The model under review builds one solid part; all positions refer to its coordinate system, in mm. Face numbers are marked on the shaded views. A direction names the side the tool comes from. Round coordinates to 2 decimals unless told otherwise and drop trailing zeros. Order: outer loops, then holes, each group sorted by start corner. A loop starts at its lowest first (then second) coordinate and runs counter-clockwise, first axis right, second up.
1) Machinability: for the marked faces 5, 6, 7 and 8, which of the approach directions +Z, -Z, +X, -X, +Y, -Y give a long, thin tool a straight path to every point of the face, cutting with its end or side? Answer none if there is none.
2) Mouldability with a two-part tool opening along Y and no side actions: class the marked faces 1, 2, 3 and 4 as pulls with the +Y half, pulls with the -Y half, needs draft (parallel to the pull), parting line crosses it, or undercut.
3) Consider section C-C (z = 2). Give the number of separate pieces and of enclosed holes in the cut face, then the cut area to 3 significant figures.
4) Consider section A-A (x = 1.5). Give the boundary of the cut face in (y, z).
5) Clearance check with flat-ended pins moving along their axes: P1, Ø1.1, axis at x = -19, z = 2.5, coming from the +Y side; P2, Ø1.5, axis at x = 14, z = 3, coming from the +Y side; P3, Ø2, axis at x = 0, z = 2, coming from the -Y side. State where each tip first meets the part, or that it passes through.
6) Consider section D-D (y = -15). Give the boundary of the cut face in (x, z).
7) To check wall thickness, follow L1, parallel to X at y = -2, z = 1.2; L2, parallel to Y at x = 16.5, z = 2.3; L3, parallel to Y at x = -16.5, z = 0.65. State the ranges of each line that lie inside material, in increasing order.
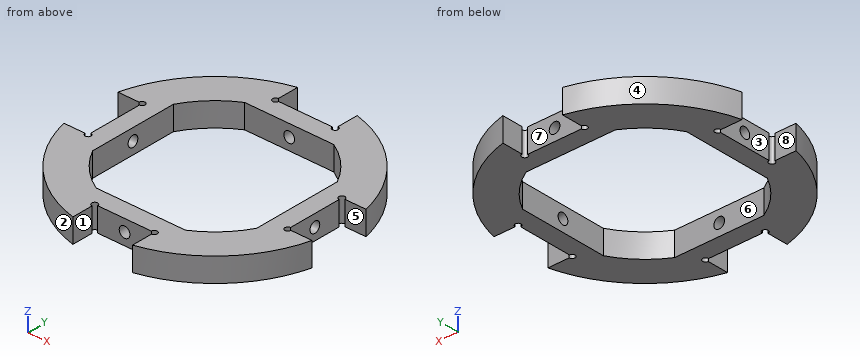
from build123d import *

# Parameters (mm, degrees)
EXTRUDE_1_DEPTH          = 4
SKETCH_2_R               = 0.9
CUT_EXTRUDE_1_DEPTH      = 43
PATTERN_CIRCULAR_1_COUNT = 4


with BuildPart() as part:
    # 草图1 → 凸台-拉伸1 (new body)
    with BuildSketch(Plane.XY):
        with BuildLine():
            Line((-4.5, 16.75), (4.5, 16.75))
            ThreePointArc((4.5, 16.75), (5.353553391, 16.396446609), (5, 17.25))
            Line((5, 17.25), (5, 20.807690886))
            ThreePointArc((5, 20.807690886), (15.132085117, 15.132085117), (20.807690886, 5))
            Line((20.807690886, 5), (17.25, 5))
            ThreePointArc((17.25, 5), (16.396446609, 5.353553391), (16.75, 4.5))
            Line((16.75, 4.5), (16.75, -4.5))
            ThreePointArc((16.75, -4.5), (16.396446609, -5.353553391), (17.25, -5))
            Line((17.25, -5), (20.807690886, -5))
            ThreePointArc((20.807690886, -5), (15.132085117, -15.132085117), (5, -20.807690886))
            Line((5, -20.807690886), (5, -17.25))
            ThreePointArc((5, -17.25), (5.353553391, -16.396446609), (4.5, -16.75))
            Line((4.5, -16.75), (-4.5, -16.75))
            ThreePointArc((-4.5, -16.75), (-5.353553391, -16.396446609), (-5, -17.25))
            Line((-5, -17.25), (-5, -20.807690886))
            ThreePointArc((-5, -20.807690886), (-15.132085117, -15.132085117), (-20.807690886, -5))
            Line((-20.807690886, -5), (-17.25, -5))
            ThreePointArc((-17.25, -5), (-16.396446609, -5.353553391), (-16.75, -4.5))
            Line((-16.75, -4.5), (-16.75, 4.5))
            ThreePointArc((-16.75, 4.5), (-16.396446609, 5.353553391), (-17.25, 5))
            Line((-17.25, 5), (-20.807690886, 5))
            ThreePointArc((-20.807690886, 5), (-15.132085117, 15.132085117), (-5, 20.807690886))
            Line((-5, 20.807690886), (-5, 17.25))
            ThreePointArc((-5, 17.25), (-5.353553391, 16.396446609), (-4.5, 16.75))
        make_face()
        with BuildLine():
            Line((-7.473954776, -13.75), (7.473954776, -13.75))
            ThreePointArc((7.473954776, -13.75), (11.066221126, -11.066221126), (13.75, -7.473954776))
            Line((13.75, -7.473954776), (13.75, 7.473954776))
            ThreePointArc((13.75, 7.473954776), (11.066221126, 11.066221126), (7.473954776, 13.75))
            Line((7.473954776, 13.75), (-7.473954776, 13.75))
            ThreePointArc((-7.473954776, 13.75), (-11.066221126, 11.066221126), (-13.75, 7.473954776))
            Line((-13.75, 7.473954776), (-13.75, -7.473954776))
            ThreePointArc((-13.75, -7.473954776), (-11.066221126, -11.066221126), (-7.473954776, -13.75))
        make_face(mode=Mode.SUBTRACT)
    extrude(amount=EXTRUDE_1_DEPTH)

    # 草图2 → 切除-拉伸1 (cut)
    with BuildSketch(Plane(origin=(0, 16.75, 0), x_dir=(1, 0, 0), z_dir=(0, 1, 0))):
        with Locations(Location((0, -2, 0), (0, 0, 180))):
            Circle(SKETCH_2_R)
    cut_extrude_1 = extrude(amount=-CUT_EXTRUDE_1_DEPTH, mode=Mode.SUBTRACT)

    # 阵列(圆周)1: 切除-拉伸1 ×4 about axis
    pattern_circular_1_axis = Axis((0, 0, 4), (0, 0, -1))
    for i in range(1, PATTERN_CIRCULAR_1_COUNT):
        add(cut_extrude_1.rotate(pattern_circular_1_axis, i * 360 / PATTERN_CIRCULAR_1_COUNT), mode=Mode.SUBTRACT)


solid = part.part
Answer below:
1. face 5: +Z, -Z, +X
1. face 6: +Z, -Z
1. face 7: +Z, -Z, +Y
1. face 8: +Z, -Z, -X
2. face 1: needs draft
2. face 2: pulls with the -Y half
2. face 3: undercut
2. face 4: pulls with the +Y half
3. separate pieces: 4
3. enclosed holes: 0
3. area: 542 mm2
4. outline: (-16.75, 0) - (-13.75, 0) - (-13.75, 4) - (-16.75, 4) - close; (13.75, 0) - (16.75, 0) - (16.75, 4) - (13.75, 4) - close
5. P1: stops at y = 10.84
5. P2: stops at y = 16.8
5. P3: stops at y = -16.75
6. outline: (-15.26, 0) - (15.26, 0) - (15.26, 4) - (-15.26, 4) - close; hole circle Ø1.8 at (0, 2)
7. L1: x = -16.75 to -13.75, 13.75 to 16.75
7. L2: y = -13.63 to -5.43, -4.57 to -0.85, 0.85 to 4.57, 5.43 to 13.63
7. L3: y = -13.63 to -5.43, -4.57 to 4.57, 5.43 to 13.63
